Source: three-view drawing plus pictorial views. Frame: mm from the lowest corner of the part. A direction names the side the tool comes from. Coordinates: 2 decimals unless noted, no trailing zeros. Write each loop counter-clockwise with the first axis right and the second up, starting at its lowest first coordinate (ties: lowest second). Pieces come first, ordered by that corner, then holes. Notation, with made-up numbers: (50.25, 70.25) -> (97.25, 70.25) arc R19 cw to (97.25, 104.25) -> close; hole circle Ø9 at (63, -31). An arc over 180 degrees is marked (long way). Write item = value, one per line.
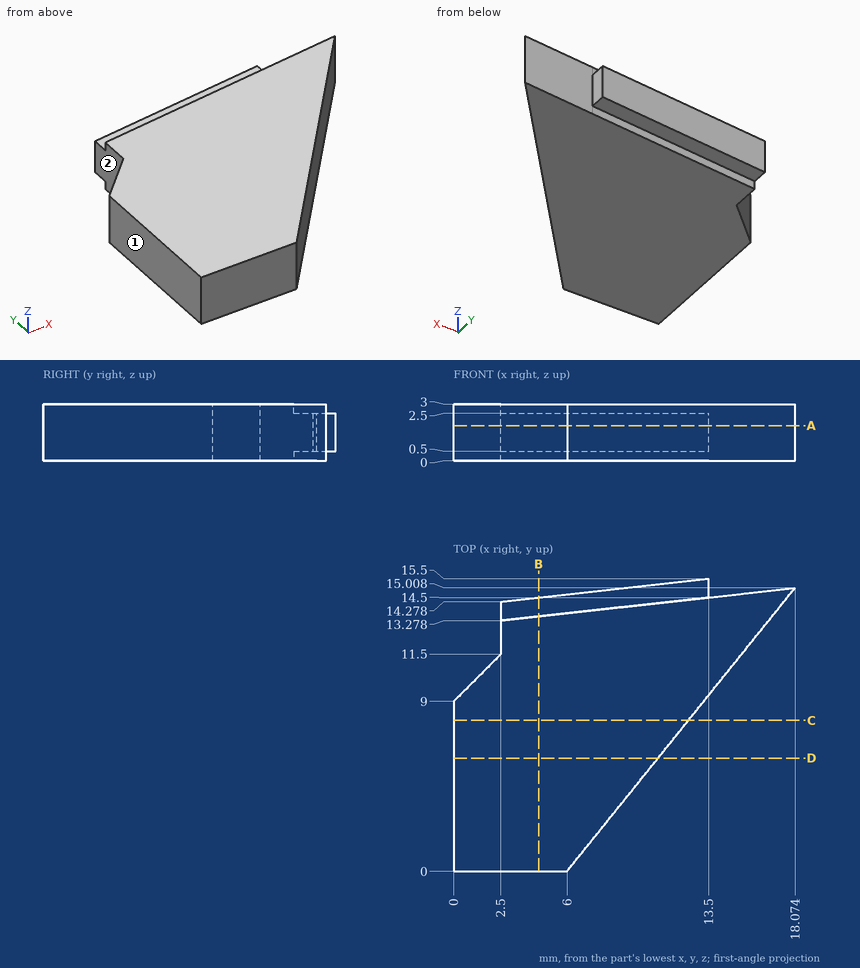
1) First-contact query: pin 1 Ø1.1 at (x, y) = (7.5, 15) entering from -Z; pin 2 Ø1.5 at (y, z) = (11.5, 0.5) entering from +X (1 decimal); pin 3 Ø1.4 at (y, z) = (13, 1.5) entering from -X. Flat tips, straight axial feed; report the tip coordinate or a pass-through.
Answer block:
pin_1 = 0.5
pin_2 = 15.9
pin_3 = 2.5
2) Cut plane A-A, the plane z = 1.85. Output: boundary loops of the cut face in (x, y), and give its area (3 significant figures).
Answer block:
outline = (0, 0) -> (6, 0) -> (18.07, 15.01) -> (13.5, 14.5) -> (13.5, 15.5) -> (2.5, 14.28) -> (2.5, 11.5) -> (0, 9) -> close
area = 166 mm2
3) Material intervals for probe 1 along X at (y, z) = (13, 0.6); probe 2 along Y at (x, z) = (17, 0.9) (1 decimal); probe 3 along Y at (x, z) = (10.5, 2.7) (1 decimal), sorted ascending. Write a range as [from, to].
Answer block:
probe_1 = [2.5, 16.46]
probe_2 = [13.7, 14.9]
probe_3 = [5.6, 14.2]
4) Reachability of the marked faces 1 and 2 from +Z, -Z, +X, -X, +Y, -Y: full face, straight path, thin tool, end or side. Return the list, or none.
Answer block:
face_1 = +Z, -Z, -X, +Y, -Y
face_2 = +Z, -Z, -X, +Y
5) Cut plane D-D, the plane y = 6. Output: boundary loops of the cut face in (x, z).
Answer block:
outline = (0, 0) -> (10.83, 0) -> (10.83, 3) -> (0, 3) -> close
6) Cut plane C-C, the plane y = 8. Output: boundary loops of the cut face in (x, z) (1 decimal).
Answer block:
outline = (0, 0) -> (12.4, 0) -> (12.4, 3) -> (0, 3) -> close
7) Cut plane B-B, the plane x = 4.5. Output: boundary loops of the cut face in (y, z), and give its area (3 significant figures).
Answer block:
outline = (0, 0) -> (13.5, 0) -> (13.5, 0.5) -> (14.5, 0.5) -> (14.5, 2.5) -> (13.5, 2.5) -> (13.5, 3) -> (0, 3) -> close
area = 42.5 mm2
